from build123d import *

# Parameters (mm, degrees)
BOSS_EXTRUDE1_DEPTH = 25
SKETCH2_R           = 3
CUT_EXTRUDE1_DEPTH  = 15
SKETCH3_R           = 3
CUT_EXTRUDE2_DEPTH  = 15
BOSS_EXTRUDE2_DEPTH = 12
BOSS_EXTRUDE4_DEPTH = 1.5
SKETCH6_R           = 4.85
CUT_EXTRUDE3_DEPTH  = 9
SKETCH7_W           = 8
SKETCH7_H           = 7.5
BOSS_EXTRUDE5_DEPTH = 4
SKETCH8_R           = 1.6
CUT_EXTRUDE4_DEPTH  = 4


with BuildPart() as part:
    # Sketch1 → Boss-Extrude1 (new body)
    with BuildSketch(Plane.XY):
        Polygon((227.088719843, 62.282971172), (227.088719843, 57.379571172), (225.590119843, 57.379571172), (225.590119843, 51.299571172), (227.088719843, 51.299571172), (227.088719843, 44.429550862), (220.178702595, 44.429550862), (220.178702595, 45.917195068), (214.098687419, 45.917195068), (214.098687419, 44.429550862), (209.19527518, 44.429550862), (209.19527518, 41.429550862), (230.088719843, 41.429550862), (230.088719843, 62.282971172), align=None)
    extrude(amount=-BOSS_EXTRUDE1_DEPTH)

    # Sketch2 → Cut-Extrude1 (cut)
    with BuildSketch(Plane(origin=(230.088719843, 0, 0), x_dir=(0, 0, -1), z_dir=(1, 0, 0))):
        with Locations((6, 54.339571172)):
            Circle(SKETCH2_R)
    extrude(amount=-CUT_EXTRUDE1_DEPTH, mode=Mode.SUBTRACT)

    # Sketch3 → Cut-Extrude2 (cut)
    with BuildSketch(Plane.XZ.offset(-41.429550862)):
        with Locations((217.138695007, -6)):
            Circle(SKETCH3_R)
    extrude(amount=-CUT_EXTRUDE2_DEPTH, mode=Mode.SUBTRACT)

    # Sketch4 → Boss-Extrude2 (add)
    with BuildSketch(Plane(origin=(0, 0, -25), x_dir=(-1, 0, 0), z_dir=(0, 0, -1))):
        with BuildLine():
            Line((-230.088719843, 62.282971172), (-234.088719843, 58.269609721))
            Line((-234.088719843, 58.269609721), (-234.088719843, 44.269609721))
            Line((-234.088719843, 44.269609721), (-242.088719843, 44.269609721))
            Line((-242.088719843, 44.269609721), (-243.840170155, 37.408191323))
            ThreePointArc((-243.840170155, 37.408191323), (-240.951322195, 29.07698458), (-232.154834185, 28.463594817))
            Line((-232.154834185, 28.463594817), (-209.19527518, 41.429550862))
            Line((-209.19527518, 41.429550862), (-230.088719843, 41.429550862))
            Line((-230.088719843, 41.429550862), (-230.088719843, 62.282971172))
        make_face()
    extrude(amount=-BOSS_EXTRUDE2_DEPTH)

    # Sketch5 → Boss-Extrude4 (add, symmetric)
    with BuildSketch(Plane(origin=(150.295838672, 132.167186427, 0), x_dir=(0.660365554, -0.750944296, 0), z_dir=(-0.750944296, -0.660365554, 0))):
        Polygon((120.831380003, -13), (134.831380003, -13), (120.831380003, 0), (116.597450455, 0), (116.597450455, -13), align=None)
    extrude(amount=BOSS_EXTRUDE4_DEPTH, both=True)

    # Sketch6 → Cut-Extrude3 (cut)
    with BuildSketch(Plane(origin=(0, 0, -25), x_dir=(-1, 0, 0), z_dir=(0, 0, -1))):
        with Locations((-236.088719843, 35.429550862)):
            Circle(SKETCH6_R)
    extrude(amount=-CUT_EXTRUDE3_DEPTH, mode=Mode.SUBTRACT)

    # Sketch7 → Boss-Extrude5 (add)
    with BuildSketch(Plane.XY.offset(-13)):
        with Locations((238.088719843, 48.019609721)):
            Rectangle(SKETCH7_W, SKETCH7_H)
    extrude(amount=-BOSS_EXTRUDE5_DEPTH)

    # Sketch8 → Cut-Extrude4 (cut)
    with BuildSketch(Plane.XY.offset(-13)):
        with Locations((238.088719843, 48.019609721)):
            Circle(SKETCH8_R)
    extrude(amount=-CUT_EXTRUDE4_DEPTH, mode=Mode.SUBTRACT)


solid = part.part
Geometry: final body of the model. Coordinates: model frame, mm. A direction names the side the tool comes from. Give positions to 0.01 mm unless a question says otherwise; leave off trailing zeros. Loops run counter-clockwise (first coordinate to the right, second up) from the corner with the lowest first, then second, coordinate; pieces in that order, holes last. Notation, with made-up numbers: (27, 21) - (79, 21) arc R18 ccw to (79, 26) - close; hole circle Ø6 at (5.25, 74). An arc over 180 degrees is marked (long way). Answer as CSV lines item,"result". Start each with the question number.
1. Section D-D, the plane z = -15.5. Return loops of the section in (x, y).
2. Draft query along Y for faces 1 (the face through (226, 57.38, -12)), 2 (the face through (220.836, 34.856, -19.084)), 3 (the face through (231.61, 33.57, -20.56)). Return one class per face: released by +Y, released by -Y, zero draft, split by the parting line, or undercut.
3. Pin query (flat end, axial travel): P1, Ø8, axis at x = 236, z = -21.5, coming from the +Y side; P2, Ø1.8, axis at x = 216.5, z = -13, coming from the +Y side; P3, Ø6, axis at y = 44, z = -16, coming from the +X side; P4, Ø5, axis at y = 54.34, z = -6, coming from the -X side. Return the tip coordinate at first contact, or that it passes through.
4. Reachability of faces 4 (the face through (238, 44.27, -21)), 5 (the face through (220.179, 45, -12)), 6 (the face through (234, 41, -13)) from +Z, -Z, +X, -X, +Y, -Y: full face, straight path, thin tool, end or side. Return the list, or none.
5. Section A-A, the plane x = 217.5. Return loops of the section in (y, z), plus the area to 3 significant figures.
6. Section C-C, the plane y = 56. Return loops of the section in (x, z).
7. Ray query, L1, parallel to X at y = 45, z = -2.75; L2, parallel to X at y = 47.5, z = -9.5; L3, parallel to Z at x = 240.5, y = 43.5. Return the intervals inside material, ascending.
8. Section B-B, the plane z = -6. Give the number of separate pieces and of enclosed holes in the cut face, plus the area to 3 significant figures.
Answers:
1,outline,"(209.2, 41.43) - (232.15, 28.46) arc R8 ccw to (243.84, 37.41) - (242.09, 44.27) - (242.09, 51.77) - (234.09, 51.77) - (234.09, 58.27) - (230.09, 62.28) - (227.09, 62.28) - (227.09, 57.38) - (225.59, 57.38) - (225.59, 51.3) - (227.09, 51.3) - (227.09, 44.43) - (220.18, 44.43) - (220.18, 45.92) - (214.1, 45.92) - (214.1, 44.43) - (209.2, 44.43) - close; hole circle Ø3.2 at (238.09, 48.02)"
2,face 1,"released by +Y"
2,face 2,"released by -Y"
2,face 3,"undercut"
3,P1,"stops at y = 60.37"
3,P2,"stops at y = 45.92"
3,P3,"stops at x = 242.92"
3,P4,"passes through"
4,face 4,"-Z, +X, +Y"
4,face 5,"+Z, -Z, +Y"
4,face 6,"+Z"
5,outline,"(36.74, -25) - (45.92, -25) - (45.92, -8.98) - (41.43, -8.98) - (41.43, -13) - (36.74, -13) - close; (41.43, -3.02) - (45.92, -3.02) - (45.92, 0) - (41.43, 0) - close"
5,area,"142 mm2"
6,outline,"(225.59, -25) - (234.09, -25) - (234.09, -13) - (230.09, -13) - (230.09, -8.5) - (225.59, -8.5) - close; (225.59, -3.5) - (230.09, -3.5) - (230.09, 0) - (225.59, 0) - close"
7,L1,"x = 214.1 to 220.18, 227.09 to 230.09"
7,L2,"x = 227.09 to 230.09"
7,L3,"z = -25 to -13"
8,separate pieces,"3"
8,enclosed holes,"0"
8,area,"102 mm2"
